```python
from build123d import *

# Parameters (mm, degrees)
RESSALTO_EXTRUS_O1_DEPTH = 25
CORTE_EXTRUS_O1_DEPTH    = 116.866302263
CORTE_EXTRUS_O2_DEPTH    = 10
CORTE_EXTRUS_O3_DEPTH    = 10
ESBO_O8_W                = 10
ESBO_O8_H                = 5
CORTE_EXTRUS_O4_DEPTH    = 108.61621625
ESBO_O10_R               = 7
CORTE_EXTRUS_O5_DEPTH    = 115.127122105
ESBO_O11_R               = 7
CORTE_EXTRUS_O6_DEPTH    = 115.127122105


with BuildPart() as part:
    # Esboço1 → Ressalto-extrusão1 (new body)
    with BuildSketch(Plane(origin=(0, 0, 0), x_dir=(1, 0, 0), z_dir=(0, 1, 0))):
        with BuildLine():
            Line((0, 0), (40, 0))
            ThreePointArc((40, 0), (80, 40), (40, 80))
            Line((40, 80), (0, 80))
            ThreePointArc((0, 80), (-40, 40), (0, 0))
        make_face()
    extrude(amount=RESSALTO_EXTRUS_O1_DEPTH)

    # Esboço5 → Corte-extrusão1 (cut, through all)
    with BuildSketch(Plane.XY):
        with BuildLine():
            Line((12.5, 25), (12.5, 14.154597668))
            ThreePointArc((12.5, 14.154597668), (20, 6.654597668), (27.5, 14.154597668))
            Line((27.5, 14.154597668), (27.5, 25))
            Line((27.5, 25), (12.5, 25))
        make_face()
    extrude(amount=-CORTE_EXTRUS_O1_DEPTH, mode=Mode.SUBTRACT)

    # Esboço6 → Corte-extrusão2 (cut)
    with BuildSketch(Plane(origin=(0, 25, 0), x_dir=(1, 0, 0), z_dir=(0, 1, 0))):
        with BuildLine():
            Line((12.5, 75), (0, 75))
            ThreePointArc((0, 75), (-35, 40), (0, 5))
            Line((0, 5), (12.5, 5))
            Line((12.5, 5), (12.5, 75))
        make_face()
    extrude(amount=-CORTE_EXTRUS_O2_DEPTH, mode=Mode.SUBTRACT)

    # Esboço7 → Corte-extrusão3 (cut)
    with BuildSketch(Plane(origin=(0, 25, 0), x_dir=(1, 0, 0), z_dir=(0, 1, 0))):
        with BuildLine():
            Line((27.5, 75), (40, 75))
            ThreePointArc((40, 75), (75, 40), (40, 5))
            Line((40, 5), (27.5, 5))
            Line((27.5, 5), (27.5, 75))
        make_face()
    extrude(amount=-CORTE_EXTRUS_O3_DEPTH, mode=Mode.SUBTRACT)

    # Esboço8 → Corte-extrusão4 (cut, through all)
    with BuildSketch(Plane(origin=(12.5, 0, 0), x_dir=(0, 0, -1), z_dir=(1, 0, 0))):
        with Locations((41.323116294, 22.5)):
            Rectangle(ESBO_O8_W, ESBO_O8_H)
    extrude(amount=-CORTE_EXTRUS_O4_DEPTH, mode=Mode.SUBTRACT)

    # Esboço10 → Corte-extrusão5 (cut, through all)
    with BuildSketch(Plane(origin=(0, 15, 0), x_dir=(1, 0, 0), z_dir=(0, 1, 0))):
        with Locations(Location((0, 40.551532556, 0), (0, 0, 270))):
            Circle(ESBO_O10_R)
    extrude(amount=-CORTE_EXTRUS_O5_DEPTH, mode=Mode.SUBTRACT)

    # Esboço11 → Corte-extrusão6 (cut, through all)
    with BuildSketch(Plane(origin=(0, 15, 0), x_dir=(1, 0, 0), z_dir=(0, 1, 0))):
        with Locations(Location((40, 40.827298834, 0), (0, 0, 270))):
            Circle(ESBO_O11_R)
    extrude(amount=-CORTE_EXTRUS_O6_DEPTH, mode=Mode.SUBTRACT)


solid = part.part
```
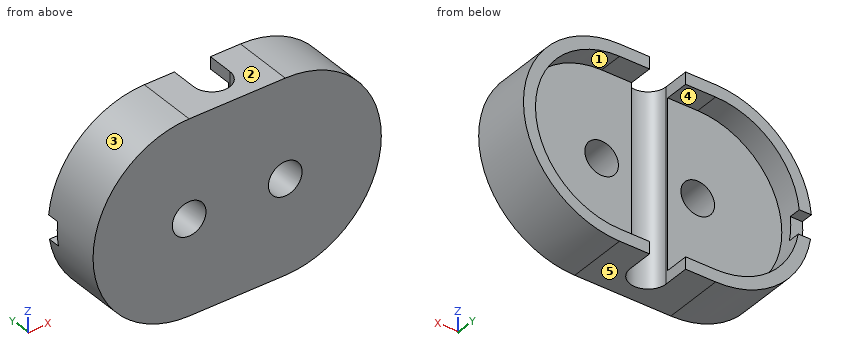
The model under review builds one solid part; all positions refer to its coordinate system, in mm. Face numbers are marked on the shaded views. A direction names the side the tool comes from. Round coordinates to 2 decimals unless told otherwise and drop trailing zeros. Loops run counter-clockwise (first coordinate to the right, second up) from the corner with the lowest first, then second, coordinate; pieces in that order, holes last. Notation, with made-up numbers: (-7.5, 1.5) - (0.5, 1.5) arc R20 cw to (0.5, 20.5) - close; hole circle Ø10 at (64, 43). An arc over 180 degrees is marked (long way). Use a Markdown table: item, result. Add a question column.
Q1. Add section A-A (y = 9.5). State the section outline as (x, z) points, plus the area to 3 significant figures.
Q2. For probe 1 along Z at (x, y) = (32, 18); probe 2 along Y at (x, z) = (37.5, -17.5); probe 3 along X at (y, z) = (9, -27), list the stretches that pass through material, from the lowest coordinate up.
Q3. The part is to be moulded in two halves that separate along X. For the marked faces 1, 2 and 3, say which applies: pulls with the +X half, pulls with the -X half, needs draft (parallel to the pull), parting line crosses it, or undercut.
Q4. Add section D-D (y = 3.75). State the section outline as (x, z) points.
Q5. Add section C-C (x = 38). State the section outline as (y, z) points.
Q6. Add section B-B (z = -40). State the section outline as (x, y) points.
Q7. Insertion check: pin 1 Ø12 at (x, y) = (-25, 13) entering from +Z; pin 2 Ø12 at (y, z) = (17, -57.5) entering from +X; pin 3 Ø12.5 at (x, z) = (40, -40.83) entering from -Y; pin 4 Ø2.5 at (x, y) = (-36, 22.5) entering from +Z. Each pin has a flat end and moves straight along its axis. Give the tip position at first contact, or say it passes through.
Q8. Machinability: for the marked faces 4 and 5, which of the approach directions +Z, -Z, +X, -X, +Y, -Y give a long, thin tool a straight path to every point of the face, cutting with its end or side? Answer none if there is none.
Worked answers:
| question | item | result |
|---|---|---|
| 1 | outline | (0, -80) - (14.12, -80) - (14.12, 0) - (0, 0) arc R40 ccw to start; (25.88, -80) - (40, -80) arc R40 ccw to (40, 0) - (25.88, 0) - close; hole circle Ø14 at (0, -40.55); hole circle Ø14 at (40, -40.83) |
| 1 | area | 6,980 mm² |
| 2 | probe 1 | -80 to -75, -5 to 0 |
| 2 | probe 2 | 0 to 15 |
| 2 | probe 3 | -37.83 to 14.55, 25.45 to 77.83 |
| 3 | face 1 | undercut |
| 3 | face 2 | needs draft |
| 3 | face 3 | pulls with the -X half |
| 4 | outline | (0, -80) - (40, -80) arc R40 ccw to (40, 0) - (0, 0) arc R40 ccw to start; hole circle Ø14 at (0, -40.55); hole circle Ø14 at (40, -40.83) |
| 5 | outline | (0, -80) - (25, -80) - (25, -75) - (15, -75) - (15, -47.54) - (0, -47.54) - close; (0, -34.12) - (15, -34.12) - (15, -5) - (25, -5) - (25, 0) - (0, 0) - close |
| 6 | outline | (-40, 0) - (-6.98, 0) - (-6.98, 15) - (-35, 15) - (-35, 20) - (-40, 20) - close; (6.98, 0) - (33.05, 0) - (33.05, 15) - (27.5, 15) - (27.5, 14.15) arc R7.5 cw to (12.5, 14.15) - (12.5, 15) - (6.98, 15) - close; (46.95, 0) - (80, 0) - (80, 25) - (75, 25) - (75, 15) - (46.95, 15) - close |
| 7 | pin 1 | z = -4.8 |
| 7 | pin 2 | x = 78.31 |
| 7 | pin 3 | through |
| 7 | pin 4 | z = -20.19 |
| 8 | face 4 | +Y |
| 8 | face 5 | -Z, +X, -X, +Y, -Y |
